from build123d import *

# Parameters (mm, degrees)
BOSS_EXTRUDE1_DEPTH = 40.56


with BuildPart() as part:
    # Sketch1 → Boss-Extrude1 (new body)
    with BuildSketch(Plane.XY):
        with BuildLine():
            ThreePointArc((182, 14.613131648), (0, 90), (-182, 14.613131648))
            Line((-182, 14.613131648), (-182, 0))
            Line((-182, 0), (-177.6, 0))
            Line((-177.6, 0), (-177.6, 4.4))
            Line((-177.6, 4.4), (-177.6, 12.781374018))
            ThreePointArc((-177.6, 12.781374018), (0, 85.6), (177.6, 12.781374018))
            Line((177.6, 12.781374018), (177.6, 4.4))
            Line((177.6, 4.4), (177.6, 0))
            Line((177.6, 0), (182, 0))
            Line((182, 0), (182, 14.613131648))
        make_face()
    extrude(amount=-BOSS_EXTRUDE1_DEPTH)


solid = part.part
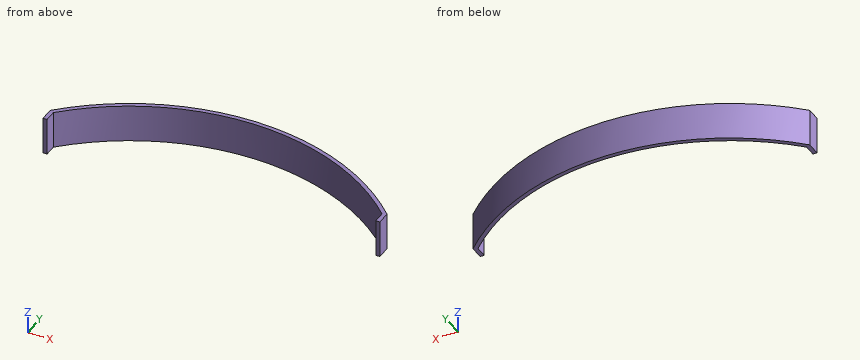
Read the model definition and answer for the solid it produces. Units are mm, in the model's axes. Coordinates: 2 decimals unless noted, no trailing zeros. Loops run counter-clockwise (first coordinate to the right, second up) from the corner with the lowest first, then second, coordinate; pieces in that order, holes last. Notation, with made-up numbers: (19.5, 11) - (64.5, 11) arc R8 cw to (64.5, 26) - close; hole circle Ø3 at (3, 45). An arc over 180 degrees is marked (long way). Answer in a Markdown table with one row per item.
Q1. Find section D-D on y = 56. Write down the section's boundary in (x, z), plus the area to 3 significant figures.
Here are the results:
| item | result |
|---|---|
| outline | (-127.85, -40.56) - (-118.75, -40.56) - (-118.75, 0) - (-127.85, 0) - close; (118.75, -40.56) - (127.85, -40.56) - (127.85, 0) - (118.75, 0) - close |
| area | 739 mm^2 |
Q2. Find section C-C on x = 24.5. Write down the section's boundary in (y, z), plus the area to 3 significant figures.
Here are the results:
| item | result |
|---|---|
| outline | (84.41, -40.56) - (88.83, -40.56) - (88.83, 0) - (84.41, 0) - close |
| area | 179 mm^2 |
Q3. Find section B-B on z = -19.5. Write down the section's boundary in (x, y), plus the area to 3 significant figures.
Here are the results:
| item | result |
|---|---|
| outline | (-182, 0) - (-177.6, 0) - (-177.6, 12.78) arc R252.99 cw to (177.6, 12.78) - (177.6, 0) - (182, 0) - (182, 14.61) arc R257.39 ccw to (-182, 14.61) - close |
| area | 1,880 mm^2 |
Q4. Straight lines are drawn through the part: line 1 along X through (y, z) = (10.5, -11); line 2 along X through (y, z) = (36, -12.5); line 3 along Y through (x, z) = (-134.5, -23). For each, find the intervals that lie inside material, in ascending order. Write a range as [from, to].
Here are the results:
| item | result |
|---|---|
| line 1 | x = [-182, -177.6], [177.6, 182] |
| line 2 | x = [-157.74, -150.45], [150.45, 157.74] |
| line 3 | y = [46.88, 52.06] |
Q5. Given P1, Ø8, axis at y = 25, z = -18.5, coming from the -X side; P2, Ø1, axis at x = 17.5, z = -9, coming from the -Y side; P3, Ø3, axis at x = 86, y = 77, coming from the +Z side; P4, Ø10, axis at y = 31, z = -22.5, coming from the -X side, each flat-ended and moving along its own axis, determine where each tip first touches the part or whether it passes through.
Here are the results:
| item | result |
|---|---|
| P1 | stops at x = -175.38 |
| P2 | stops at y = 84.96 |
| P3 | passes through |
| P4 | stops at x = -169.85 |
